For this review, take the finished solid that the model builds, in its own axes (mm). A direction names the side the tool comes from. Give positions to 0.01 mm unless a question says otherwise; leave off trailing zeros. Write each loop counter-clockwise with the first axis right and the second up, starting at its lowest first coordinate (ties: lowest second). Pieces come first, ordered by that corner, then holes.
from build123d import *

# Parameters (mm, degrees)
BOSS_EXTRUDE1_DEPTH = 8
CHAMFER2_START      = 20.859650045
CHAMFER2_OUTLINE_W  = 12
CHAMFER2_OUTLINE_H  = 7
CHAMFER2_DEPTH      = 5.140349955
CHAMFER3_START      = -26
CHAMFER3_OUTLINE_W  = 12
CHAMFER3_OUTLINE_H  = 7
CHAMFER3_DEPTH      = 5.140349955
SKETCH2_R           = 3.5
CUT_EXTRUDE1_DEPTH  = 16
SKETCH3_R           = 3.5
CUT_EXTRUDE2_DEPTH  = 49.833796009


with BuildPart() as part:
    # Sketch1 → Boss-Extrude1 (new, symmetric)
    with BuildSketch(Plane.XY):
        Polygon((-6.5, 0), (6.5, 0), (6.5, -8.404669261), (27.5, -8.404669261), (27.5, -1.404669261), (14.5, -1.404669261), (14.5, 23.595330739), (4.5, 23.595330739), (4.5, 7.159533074), (-4.5, 7.159533074), (-4.5, 23.595330739), (-14.5, 23.595330739), (-14.5, -1.404669261), (-27.5, -1.404669261), (-27.5, -8.404669261), (-6.5, -8.404669261), align=None)
    extrude(amount=BOSS_EXTRUDE1_DEPTH, both=True)

    # Chamfer2: read off the stored shape, not the designer's step
    # Chamfer2 outline → Chamfer2 (cut)
    with BuildSketch(Plane(origin=(0, 0, 0), x_dir=(0.7071067811865474, 0, -0.7071067811865477), z_dir=(0.7071067811865476, 0, 0.7071067811865476)).offset(CHAMFER2_START)):
        with Locations((14, -4.904669261)):
            Rectangle(CHAMFER2_OUTLINE_W, CHAMFER2_OUTLINE_H)
    extrude(amount=CHAMFER2_DEPTH, mode=Mode.SUBTRACT)

    # Chamfer3: read off the stored shape, not the designer's step
    # Chamfer3 outline → Chamfer3 (cut)
    with BuildSketch(Plane(origin=(0, 0, 0), x_dir=(0.707106781186548, 0, 0.707106781186547), z_dir=(0.707106781186547, 0, -0.707106781186548)).offset(CHAMFER3_START)):
        with Locations((-14, 4.904669261)):
            Rectangle(CHAMFER3_OUTLINE_W, CHAMFER3_OUTLINE_H)
    extrude(amount=CHAMFER3_DEPTH, mode=Mode.SUBTRACT)

    # Sketch2 → Cut-Extrude1 (cut)
    with BuildSketch(Plane(origin=(0, -1.404669261, 0), x_dir=(1, 0, 0), z_dir=(0, 1, 0))):
        with Locations(Location((21, 0, 0), (0, 0, 180))):
            Circle(SKETCH2_R)
    cut_extrude1 = extrude(amount=-CUT_EXTRUDE1_DEPTH, mode=Mode.SUBTRACT)

    # Mirror1: Cut-Extrude1 across plane
    add(cut_extrude1.mirror(Plane(origin=(0, 0, 0), x_dir=(0, 0, 1), z_dir=(1, 0, 0))), mode=Mode.SUBTRACT)

    # Sketch3 → Cut-Extrude2 (cut, through all)
    with BuildSketch(Plane(origin=(14.5, 0, 0), x_dir=(0, 0, -1), z_dir=(1, 0, 0))):
        with Locations((0, 15.595330739)):
            Circle(SKETCH3_R)
    extrude(amount=-CUT_EXTRUDE2_DEPTH, mode=Mode.SUBTRACT)


solid = part.part
(1) Tool access review of faces 1 (the flat face through (4.5, 15, 4)), 2 (the flat face through (6.5, -4, 0)), 3 (the flat face through (14.5, 11, 0)): name each direction out of +Z, -Z, +X, -X, +Y, -Y from which nothing blocks a thin tool from reaching the whole face with its end or side.
(2) We need section D-D (z = 4.5). Write out the cut boundary in (x, y).
(3) For L1, parallel to Z at x = -21, y = -4.25; L2, parallel to Y at x = -9.25, z = 0; L3, parallel to X at y = 14.5, z = 7, list the stretches that pass through material, from the lowest coordinate up.
(4) We need section B-B (y = -4.5). Write out the cut boundary in (x, z).
(5) The part is to be moulded in two halves that separate along Z. For faces 4 (the cylindrical face through (9.57, 12.18, 0.76)), 5 (the flat face through (-24.5, -5, 5)), 6 (the flat face through (19.6, -1.405, -3.4)), 7 (the cylindrical face through (17.66, -4.86, 1.05)), say which applies: +Z half, -Z half, draft (parallel to the pull), parting line (faces both ways), or undercut.
(6) We need section A-A (z = 0). Count the separate pieces of the cut face and the enclosed holes in it, and give its area (3 significant figures).
(7) We need section C-C (y = 21.5). Write out the cut boundary in (x, z), and give its area (3 significant figures).
(8) Clearance check with flat-ended pins moving along their axes: pin 1 Ø8 at (y, z) = (15.6, 0) entering from +X; pin 2 Ø6.5 at (x, z) = (21.5, -1.5) entering from +Y; pin 3 Ø8 at (x, z) = (21, 0) entering from -Y; pin 4 Ø6.5 at (x, z) = (-1, -3) entering from -Y. State where each tip first meets the part, or that it passes through.
The answers:
1. face 1: +Z, -Z, +Y
1. face 2: +Z, -Z, -Y
1. face 3: +Z, -Z, +X, +Y
2. outline: (-25, -8.4) - (-6.5, -8.4) - (-6.5, 0) - (6.5, 0) - (6.5, -8.4) - (25, -8.4) - (25, -1.4) - (14.5, -1.4) - (14.5, 23.6) - (4.5, 23.6) - (4.5, 7.16) - (-4.5, 7.16) - (-4.5, 23.6) - (-14.5, 23.6) - (-14.5, -1.4) - (-25, -1.4) - close
3. L1: z = -8 to -3.5, 3.5 to 8
3. L2: y = -8.4 to 12.1, 19.1 to 23.6
3. L3: x = -14.5 to -4.5, 4.5 to 14.5
4. outline: (-27.5, -8) - (-6.5, -8) - (-6.5, 8) - (-21.5, 8) - (-27.5, 2) - close; (6.5, -8) - (27.5, -8) - (27.5, 2) - (21.5, 8) - (6.5, 8) - close; hole circle Ø7 at (-21, 0); hole circle Ø7 at (21, 0)
5. face 4: undercut
5. face 5: +Z half
5. face 6: draft
5. face 7: undercut
6. separate pieces: 5
6. enclosed holes: 0
6. area: 615 mm2
7. outline: (-14.5, -8) - (-4.5, -8) - (-4.5, 8) - (-14.5, 8) - close; (4.5, -8) - (14.5, -8) - (14.5, 8) - (4.5, 8) - close
7. area: 320 mm2
8. pin 1: stops at x = 14.5
8. pin 2: stops at y = -1.4
8. pin 3: stops at y = -8.4
8. pin 4: stops at y = 0
